Geometry: see drawing. Coordinates: mm, zero at the bounding-box minimum. Round coordinates to 2 decimals unless told otherwise and drop trailing zeros. Order: outer loops, then holes, each group sorted by start corner. A loop starts at its lowest first (then second) coordinate and runs counter-clockwise, first axis right, second up. Notation, with made-up numbers: M -33.75,87.25 L -16.75,87.25 A16 cw -16.75,115.25 Z; hole C -10,15 d6. An arc over 180 degrees is marked long. Answer in a Markdown table with one row per item. Add a question column.
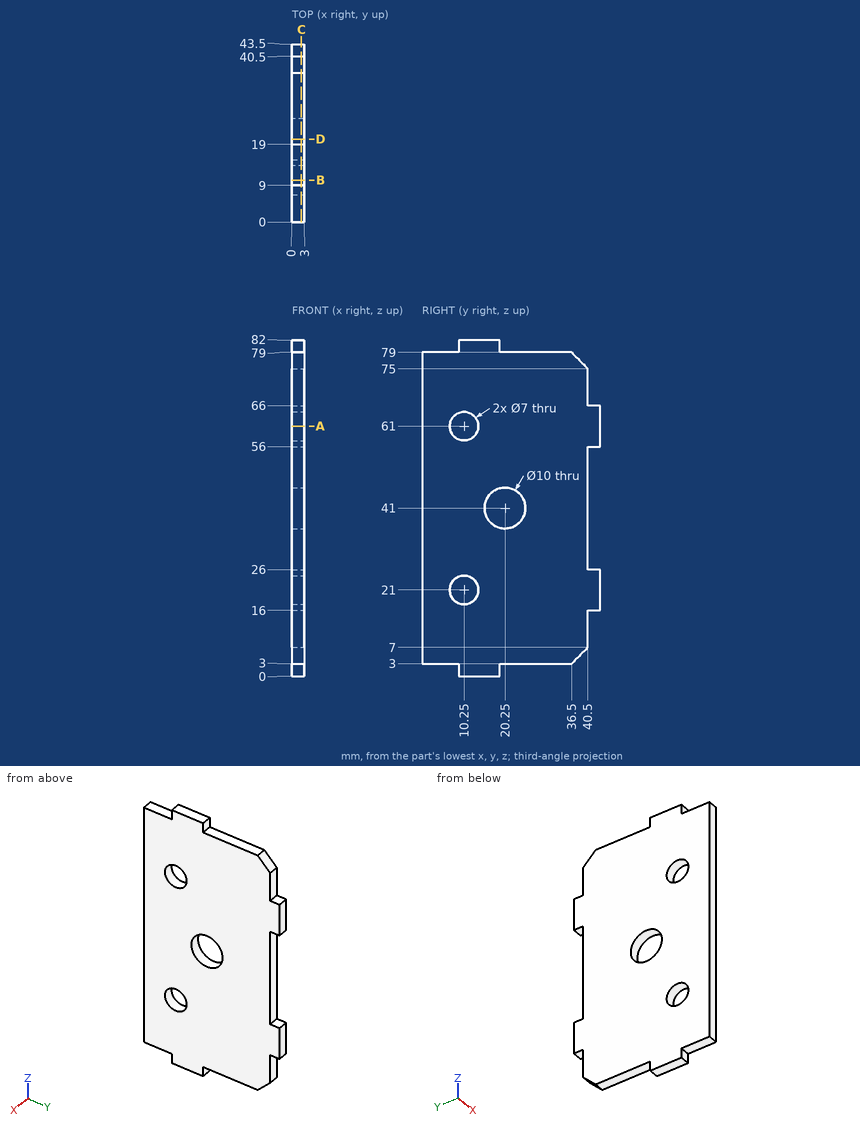
(1) Cut plane D-D (y = 20.25). Return loops of the section in (x, z), and give its area (3 significant figures).
(2) Cut plane C-C (x = 2.35). Return loops of the section in (y, z), and give its area (3 significant figures).
(3) Line query: line 1 (Z direction, x = 2.15, y = 10.25); line 2 (Y direction, x = 1.55, z = 21); line 3 (Z direction, x = 0.15, y = 41.5). Output: solid intervals per line, ascending. Write a range as from..to.
(4) Cut plane B-B (y = 10.25). Return loops of the section in (x, z), and give its area (3 significant figures).
(5) Pin query (flat end, axial travel): pin 1 (1.5 mm diameter, centred on x = 1.5, z = 43, fed in from +Y); pin 2 (4 mm diameter, centred on y = 10.25, z = 61, fed in from -X); pin 3 (0.9 mm diameter, centred on x = 1.5, y = 42, fed in from +Z); pin 4 (1.5 mm diameter, centred on x = 2, z = 27.5, fed in from -Y). Return the tip coordinate at first contact, or that it passes through.
(6) Cut plane A-A (z = 61). Return loops of the section in (x, y), and give its area (4 significant figures).
Answer list:
| question | item | result |
|---|---|---|
| 1 | outline | M 0,3 L 3,3 L 3,36 L 0,36 Z; M 0,46 L 3,46 L 3,79 L 0,79 Z |
| 1 | area | 198 mm² |
| 2 | outline | M 0,3 L 9,3 L 9,0 L 19,0 L 19,3 L 36.5,3 L 40.5,7 L 40.5,16 L 43.5,16 L 43.5,26 L 40.5,26 L 40.5,56 L 43.5,56 L 43.5,66 L 40.5,66 L 40.5,75 L 36.5,79 L 19,79 L 19,82 L 9,82 L 9,79 L 0,79 Z; hole C 10.25,21 d7; hole C 10.25,61 d7; hole C 20.25,41 d10 |
| 2 | area | 3,030 mm² |
| 3 | line 1 | 0..17.5, 24.5..57.5, 64.5..82 |
| 3 | line 2 | 0..6.75, 13.75..43.5 |
| 3 | line 3 | 16..26, 56..66 |
| 4 | outline | M 0,0 L 3,0 L 3,17.5 L 0,17.5 Z; M 0,24.5 L 3,24.5 L 3,57.5 L 0,57.5 Z; M 0,64.5 L 3,64.5 L 3,82 L 0,82 Z |
| 4 | area | 204 mm² |
| 5 | pin 1 | y = 40.5 |
| 5 | pin 2 | through |
| 5 | pin 3 | z = 66 |
| 5 | pin 4 | y = 0 |
| 6 | outline | M 0,0 L 3,0 L 3,6.75 L 0,6.75 Z; M 0,13.75 L 3,13.75 L 3,43.5 L 0,43.5 Z |
| 6 | area | 109.5 mm² |
